Source: three-view drawing plus pictorial views. Frame: mm from the lowest corner of the part. A direction names the side the tool comes from. Round coordinates to 2 decimals unless told otherwise and drop trailing zeros. Write each loop counter-clockwise with the first axis right and the second up, starting at its lowest first coordinate (ties: lowest second). Pieces come first, ordered by that corner, then holes. Notation, with made-up numbers: M 83.25,20 L 123.25,20 A18 ccw 123.25,37 Z; hole C -14.75,-8 d6. An arc over 180 degrees is marked long. Put each result on its own line as item: value. Start each with the question number.
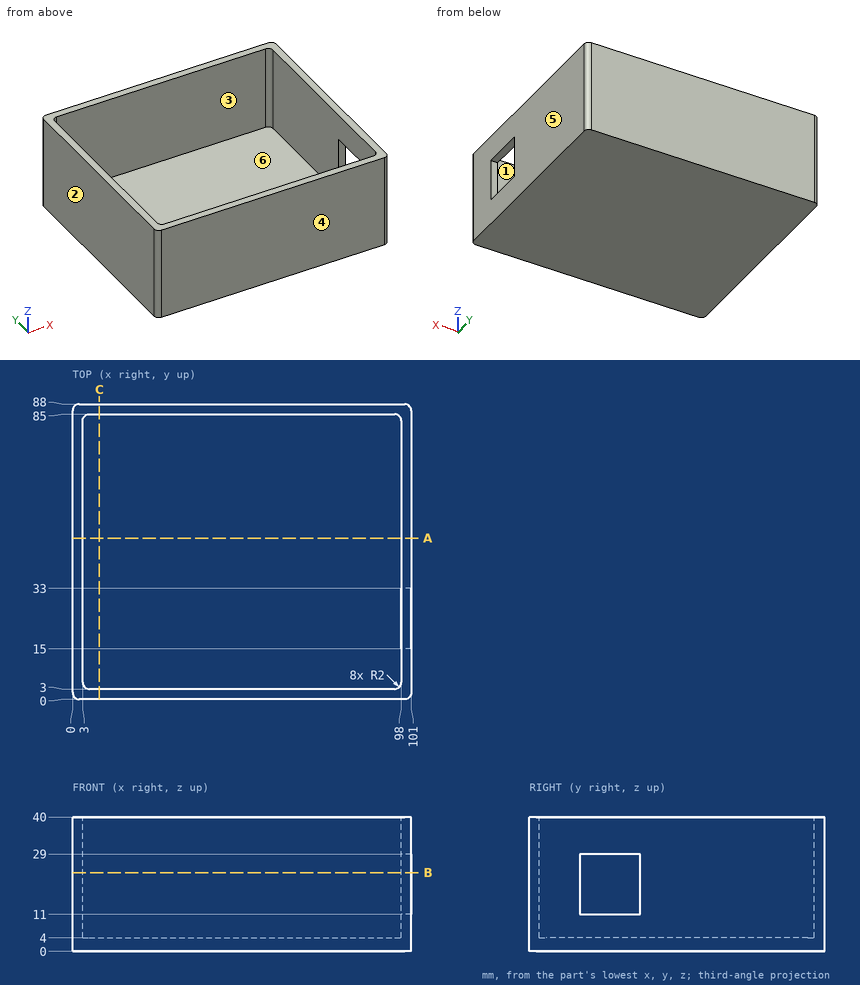
(1) Section query A-A (y = 48). Return loops of the section in (x, z), and give its area (3 significant figures).
(2) Section query C-C (x = 8). Return loops of the section in (y, z).
(3) Ray query, line 1 along Y through (x, z) = (72, 22); line 2 along X through (y, z) = (8.5, 4.5); line 3 along Z through (x, y) = (93, 73). Return the intervals inside material, ascending.
(4) Contact query for a flat-ended pin moving along its axis: P1, Ø24.5, axis at x = 55.5, y = 39.5, coming from the +Z side. Output: stop coordinate, or through.
(5) Access query for the marked faces 1 and 2. Directions: +Z, -Z, +X, -X, +Y, -Y. A direction counts if a zero-diameter tool reaches every point of the face in a straight line with its end or side. Return the directions, or none.
(6) Section query B-B (z = 23.5). Return loops of the section in (x, y), and give its area (3 significant figures).
(7) Pull-direction query (X, two-part tool) for the marked faces 3, 4, 5 and 6; classes: +X half, -X half, draft (parallel to the pull), parting line (faces both ways), or undercut.
Entries:
1. outline: M 0,0 L 101,0 L 101,40 L 98,40 L 98,4 L 3,4 L 3,40 L 0,40 Z
1. area: 620 mm2
2. outline: M 0,0 L 88,0 L 88,40 L 85,40 L 85,4 L 3,4 L 3,40 L 0,40 Z
3. line 1: 0 to 3, 85 to 88
3. line 2: 0 to 3, 98 to 101
3. line 3: 0 to 4
4. P1: z = 4
5. face 1: +Z
5. face 2: +Z, -Z, -X, +Y, -Y
6. outline: M 0,2 A2 ccw 2,0 L 99,0 A2 ccw 101,2 L 101,15 L 98,15 L 98,5 A2 cw 96,3 L 5,3 A2 cw 3,5 L 3,83 A2 cw 5,85 L 96,85 A2 cw 98,83 L 98,33 L 101,33 L 101,86 A2 ccw 99,88 L 2,88 A2 ccw 0,86 Z
6. area: 1,040 mm2
7. face 3: undercut
7. face 4: draft
7. face 5: +X half
7. face 6: undercut
